```python
from build123d import *

# Parameters (mm, degrees)
SKETCH1_R           = 1.5
SKETCH1_R_2         = 1
SKETCH1_R_3         = 2
BOSS_EXTRUDE1_DEPTH = 4.5
FILLET1_R           = 10


with BuildPart() as part:
    # Sketch1 → Boss-Extrude1 (new body)
    with BuildSketch(Plane(origin=(0, 0, 0), x_dir=(1, 0, 0), z_dir=(0, 1, 0))):
        with BuildLine():
            ThreePointArc((-6.456463654, -0.468407199), (-5.880915222, -3.152272765), (-4.357266756, -5.43544725))
            Line((-4.357266756, -5.43544725), (2.344258018, -10.938071213))
            ThreePointArc((2.344258018, -10.938071213), (5.202990751, -11.141955791), (6.634993867, -8.659358597))
            Line((6.634993867, -8.659358597), (6.640943349, 1.930649732))
            ThreePointArc((6.640943349, 1.930649732), (5.809058186, 9.628967625), (6.558640267, 17.335734652))
            ThreePointArc((6.558640267, 17.335734652), (6.597770339, 17.526968722), (6.637884512, 17.717998785))
            ThreePointArc((6.637884512, 17.717998785), (2.603251894, 23.964804241), (-3.96716661, 20.4819262))
            ThreePointArc((-3.96716661, 20.4819262), (-4.005352419, 20.366730432), (-4.043270963, 20.251446412))
            ThreePointArc((-4.043270963, 20.251446412), (-6.29279682, 10.012987158), (-6.456463654, -0.468407199))
        make_face()
        Circle(SKETCH1_R, mode=Mode.SUBTRACT)
        with Locations((3.64018052, -7.995416238)):
            Circle(SKETCH1_R_2, mode=Mode.SUBTRACT)
        with Locations((1.216156784, 18.642589744)):
            Circle(SKETCH1_R_3, mode=Mode.SUBTRACT)
    extrude(amount=BOSS_EXTRUDE1_DEPTH)

    # Fillet1
    fillet1_edges = [part.edges().sort_by_distance(p)[0] for p in [
        (6.640943349, 2.25, -1.930649732),
    ]]
    fillet(fillet1_edges, radius=FILLET1_R)


solid = part.part
```
The listing builds one solid part. Answer for the finished solid, in the listing's coordinates (mm). A direction names the side the tool comes from. Coordinates: 2 decimals unless noted, no trailing zeros. Write each loop counter-clockwise with the first axis right and the second up, starting at its lowest first coordinate (ties: lowest second). Pieces come first, ordered by that corner, then holes. Notation, with made-up numbers: (51.25, 80.25) - (98.25, 80.25) arc R18 cw to (98.25, 103.25) - close; hole circle Ø1 at (25, 48.5). An arc over 180 degrees is marked (long way). One line per item, written item: value.
1) A tool of negligible diameter and unlimited length cuts with its end or side. For faces 4 (the cylindrical face through (6.6, 2.28, -1.86)), 5 (the cylindrical face through (3.42, 2.22, 8.97)), from which of +Z, -Z, +X, -X, +Y, -Y can it reach the whole face along a straight path? Write none if from no direction.
Geometry check:
face 4: +X, +Y, -Y
face 5: +Y, -Y
2) Consider line 1 along Z through (x, y) = (0, 1.4); line 2 along X through (y, z) = (4.1, 7.5); line 3 along Z through (x, y) = (-1.25, 2.9). Determine where each line is inside the solid, lowest interval first. Write a range as from..to.
Geometry check:
line 1: z = -24.01..-20.23, -17.05..-1.5, 1.5..9.01
line 2: x = -1.84..2.77, 4.51..6.64
line 3: z = -23.56..-0.83, 0.83..7.99
3) Find section D-D (x = 0). Give the vertices of the cut face in (y, z), and give its area (3 significant figures).
Geometry check:
outline: (0, -24.01) - (4.5, -24.01) - (4.5, -20.23) - (0, -20.23) - close; (0, -17.05) - (4.5, -17.05) - (4.5, -1.5) - (0, -1.5) - close; (0, 1.5) - (4.5, 1.5) - (4.5, 9.01) - (0, 9.01) - close
area: 121 mm2
4) For a pull along X with two mould halves and no side action, classify faces 1 (the cylindrical face through (-1.5, 2.22, -0.07)), 2 (the flat face through (0, 4.5, -7)), 3 (the cylindrical face through (-5.896, 2.218, 3.117)) as pulls with the +X half, pulls with the -X half, needs draft (parallel to the pull), parting line crosses it, or undercut.
Geometry check:
face 1: undercut
face 2: needs draft
face 3: pulls with the -X half
5) Find section C-C (y = 2.45). Count the separate pieces of the cut face and the enclosed holes in it, and give its area (3 significant figures).
Geometry check:
separate pieces: 1
enclosed holes: 3
area: 364 mm2
6) Find section B-B (z = 0). Give the vertices of the cut face in (x, y), and give its area (3 significant figures).
Geometry check:
outline: (-6.49, 0) - (-1.5, 0) - (-1.5, 4.5) - (-6.49, 4.5) - close; (1.5, 0) - (6.64, 0) - (6.64, 4.5) - (1.5, 4.5) - close
area: 45.6 mm2
7) Find section A-A (x = 4). Give the vertices of the cut face in (y, z), and give its area (3 significant figures).
Geometry check:
outline: (0, -23.39) - (4.5, -23.39) - (4.5, 7.06) - (0, 7.06) - close; (0, 8.93) - (4.5, 8.93) - (4.5, 11.46) - (0, 11.46) - close
area: 148 mm2
8) This flat-tipped pin is pushed along its axis until it touches: pin 1 Ø1 at (x, y) = (-4, 1) entering from -Z. Where does it stop, or does it pass through?
Geometry check:
pin 1: stops at z = -21.47
